The listing builds one solid part. Answer for the finished solid, in the listing's coordinates (mm). Round coordinates to 2 decimals unless told otherwise and drop trailing zeros. Write each loop counter-clockwise with the first axis right and the second up, starting at its lowest first coordinate (ties: lowest second). Pieces come first, ordered by that corner, then holes.
from build123d import *

# Parameters (mm, degrees)
F0_R          = 15
F1_DEPTH      = 30
F2_R          = 15
F3_DEPTH      = 10
F4_DEPTH      = 25
F6_R          = 7
F7_DEPTH      = 130
F7_DEPTH_BACK = 140
F8_R          = 4
F9_DEPTH      = 10
F10_R         = 4.5
F11_DEPTH     = 15


# Not quite as in the source:
# - a pattern or mirror of a feature is missing from the dataset's text; its kind, count and spacing are read off the source's solid


with BuildPart() as f1:
    # F0 (on Top) → F1 (new body)
    with BuildSketch(Plane.XY):
        Circle(F0_R)
    extrude(amount=F1_DEPTH)

    # F2 (on face) → F3 (join)
    with BuildSketch(Plane.XY.offset(30)):
        with BuildLine():
            ThreePointArc((10.5356537529, -17), (17.4744538549, -9.7284871625), (20, 0))
            ThreePointArc((20, 0), (17.4744538549, 9.7284871625), (10.5356537529, 17))
            Line((10.5356537529, 17), (-10.5356537529, 17))
            ThreePointArc((-10.5356537529, 17), (-16.9661727605, 10.5900416364), (-19.9, 1.9974984355))
            ThreePointArc((-19.9, 1.9974984355), (-18.5508623254, 1.3784048752), (-18, 0))
            ThreePointArc((-18, 0), (-18.5508623254, -1.3784048752), (-19.9, -1.9974984355))
            ThreePointArc((-19.9, -1.9974984355), (-16.9661727605, -10.5900416364), (-10.5356537529, -17))
            Line((-10.5356537529, -17), (10.5356537529, -17))
        make_face()
        Circle(F2_R, mode=Mode.SUBTRACT)
        with BuildLine():
            ThreePointArc((10.5356537529, 17), (17.4744538549, 9.7284871625), (20, 0))
            ThreePointArc((20, 0), (17.4744538549, -9.7284871625), (10.5356537529, -17))
            Line((10.5356537529, -17), (18.3303027798, -17))
            ThreePointArc((18.3303027798, -17), (23.2729195579, -9.1307839342), (25, 0))
            ThreePointArc((25, 0), (23.2729195579, 9.1307839342), (18.3303027798, 17))
            Line((18.3303027798, 17), (10.5356537529, 17))
        make_face()
        with BuildLine():
            ThreePointArc((-19.9, 1.9974984355), (-16.9661727605, 10.5900416364), (-10.5356537529, 17))
            Line((-10.5356537529, 17), (-18.3303027798, 17))
            ThreePointArc((-18.3303027798, 17), (-25, 0), (-18.3303027798, -17))
            Line((-18.3303027798, -17), (-10.5356537529, -17))
            ThreePointArc((-10.5356537529, -17), (-16.9661727605, -10.5900416364), (-19.9, -1.9974984355))
            ThreePointArc((-19.9, -1.9974984355), (-22, 0), (-19.9, 1.9974984355))
        make_face()
        with BuildLine():
            ThreePointArc((-18, 0), (-18.5508623254, 1.3784048752), (-19.9, 1.9974984355))
            ThreePointArc((-19.9, 1.9974984355), (-20, 0), (-19.9, -1.9974984355))
            ThreePointArc((-19.9, -1.9974984355), (-18.5508623254, -1.3784048752), (-18, 0))
        make_face()
        with BuildLine():
            ThreePointArc((-19.9, -1.9974984355), (-20, 0), (-19.9, 1.9974984355))
            ThreePointArc((-19.9, 1.9974984355), (-22, 0), (-19.9, -1.9974984355))
        make_face()
        Circle(F2_R)
    extrude(amount=F3_DEPTH)

    # F2 (on face) → F4 (cut)
    with BuildSketch(Plane.XY.offset(30)):
        with BuildLine():
            ThreePointArc((-18, 0), (-18.5508623254, 1.3784048752), (-19.9, 1.9974984355))
            ThreePointArc((-19.9, 1.9974984355), (-20, 0), (-19.9, -1.9974984355))
            ThreePointArc((-19.9, -1.9974984355), (-18.5508623254, -1.3784048752), (-18, 0))
        make_face()
        with BuildLine():
            ThreePointArc((-19.9, -1.9974984355), (-20, 0), (-19.9, 1.9974984355))
            ThreePointArc((-19.9, 1.9974984355), (-22, 0), (-19.9, -1.9974984355))
        make_face()
    f4 = extrude(amount=F4_DEPTH, mode=Mode.SUBTRACT)

    # F4_copies: F4 across plane
    add(f4.mirror(Plane(origin=(0, 0, 0), x_dir=(-0.9659258263, -0.2588190451, 0), z_dir=(0.2588190451, -0.9659258263, 0))), mode=Mode.SUBTRACT)

    # F4_copies1: F4 across plane
    add(f4.mirror(Plane(origin=(0, 0, 0), x_dir=(0.9659258263, -0.2588190451, 0), z_dir=(0.2588190451, 0.9659258263, 0))), mode=Mode.SUBTRACT)

    # F4_copies2: F4 across plane
    add(f4.mirror(Plane(origin=(0, 0, 0), x_dir=(0.2588190451, 0.9659258263, 0), z_dir=(0.9659258263, -0.2588190451, 0))), mode=Mode.SUBTRACT)

    # F4_copies3: F4 across plane
    add(f4.mirror(Plane(origin=(0, 0, 0), x_dir=(-0.2588190451, 0.9659258263, 0), z_dir=(0.9659258263, 0.2588190451, 0))), mode=Mode.SUBTRACT)

    # F6 (on face) → F7 (join, two sides)
    with BuildSketch(Plane(origin=(0, 0, 0), x_dir=(1, 0, 0), z_dir=(0, 0, -1))) as f7_sk:
        Circle(F6_R)
    extrude(amount=F7_DEPTH)
    extrude(f7_sk.sketch, amount=-F7_DEPTH_BACK)

    # F8 (on face) → F9 (join)
    with BuildSketch(Plane(origin=(0, 0, -130), x_dir=(1, 0, 0), z_dir=(0, 0, -1))):
        Circle(F8_R)
    extrude(amount=F9_DEPTH)

    # F10 (on face) → F11 (join)
    with BuildSketch(Plane.XY.offset(140)):
        Circle(F10_R)
    extrude(amount=F11_DEPTH)


solid = f1.part
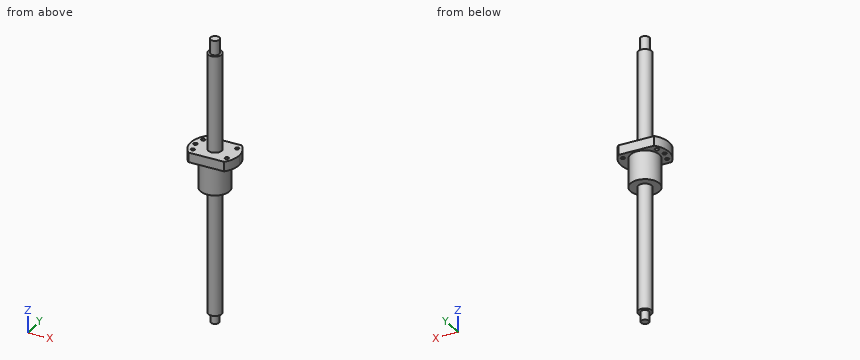
1. Given pin 1 (4 mm diameter, centred on y = 0, z = -44, fed in from -X); pin 2 (3 mm diameter, centred on x = 16, y = 6.5, fed in from +Z); pin 3 (3 mm diameter, centred on y = -7.5, z = 113, fed in from +X); pin 4 (17 mm diameter, centred on x = 10.5, y = -3.5, fed in from +Z), each flat-ended and moving along its own axis, determine where each tip first touches the part or whether it passes through.
Geometry says:
pin 1: stops at x = -7
pin 2: stops at z = 40
pin 3: stops at x = 3.61
pin 4: stops at z = 155
2. Section B-B on z = 8 is taken. Determine the outline of the cut face in (x, y), plus the area to 3 significant figures.
Geometry says:
outline: circle Ø30 at (0, 0)
area: 707 mm2
3. Straight lines are drawn through the part: line 1 along Z through (x, y) = (10, 10); line 2 along Z through (x, y) = (20, 5); line 3 along X through (y, z) = (-1, -79.5). For each, find the intervals that lie inside material, in ascending order.
Geometry says:
line 1: z = 0 to 40
line 2: z = 30 to 40
line 3: x = -6.93 to 6.93
4. Section C-C on z = 133.5 is taken. Determine the outline of the cut face in (x, y).
Geometry says:
outline: circle Ø14 at (0, 0)
5. Section A-A on x = 10.5 is taken. Determine the outline of the cut face in (y, z), plus the area to 3 significant figures.
Geometry says:
outline: (-17, 30) - (-10.71, 30) - (-10.71, 0) - (10.71, 0) - (10.71, 30) - (17, 30) - (17, 40) - (-17, 40) - close
area: 983 mm2
